Autodesk Inventor part; units mm, degrees
ref_plane "YZ Plane" through (0, 0, 0) normal (1, 0, 0) x (0, 1, 0)
ref_plane "XZ Plane" through (0, 0, 0) normal (0, 1, 0) x (-1, 0, 0)
ref_plane "XY Plane" through (0, 0, 0) normal (0, 0, 1) x (1, 0, 0)
sketch "Sketch1" plane through (0, 0, 0) normal (0, 0, 1) x (1, 0, 0)
  line L0 (0, 0) -> (6.35, 0)
  line L1 (6.35, 0) -> (6.35, 25.4)
  line L2 (6.35, 25.4) -> (0, 25.4)
  line L3 (0, 25.4) -> (0, 0)
  line L4 (6.35, 0) -> (6.35, -5.2605)
  line L5 (6.35, -5.2605) -> (12.7, -11.6105)
  line L6 (12.7, -11.6105) -> (12.7, -24.3105)
  arc A0 (12.7, -24.3105) -> (25.4, -24.3105) centre (19.05, -24.3105) ccw
  line L7 (25.4, -24.3105) -> (25.4, -6.35)
  line L8 (25.4, -6.35) -> (6.35, 12.7)
  dimension "d0" = 6.35
  dimension "d1" = 25.4
  dimension "d2" = 6.35
  dimension "d3" = 12.7
  dimension "d4" = 12.7
  dimension "d5" = 45
extrude "Extrusion1" add sketch "Sketch1" along normal blind 6.35
fillet "Fillet1" radius 3.175 1 edges at (6.35, -5.2605, 3.175)
fillet "Fillet2" radius 12.7 3 edges at (12.7, -11.6105, 3.175) (25.4, -6.35, 3.175) (6.35, 12.7, 3.175)
sketch "Sketch2" plane through (0, 0, 6.35) normal (0, 0, 1) x (1, 0, 0)
  arc A0 (12.7, -24.3105) -> (25.4, -24.3105) centre (19.05, -24.3105) ccw
hole "Hole1" at (19.05, -24.3105, 6.35) direction (0, 0, -1) diameter 6.7564 end through all
ref_plane "Work Plane1" through (11.7701, -1.7003, 6.35) normal (-0.7071, -0.7071, 0) x (-0.7071, 0.7071, 0)
properties part number "Mirror"
Work out the finished part from the listing and answer in its coordinate system (mm). A direction names the side the tool comes from. Coordinates: 2 decimals unless noted, no trailing zeros. Write each loop counter-clockwise with the first axis right and the second up, starting at its lowest first coordinate (ties: lowest second). Pieces come first, ordered by that corner, then holes.
1. Consider line 1 along Y through (x, z) = (19.05, 4.75); line 2 along Y through (x, z) = (20, 5); line 3 along X through (y, z) = (-17, 2). Determine where each line is inside the solid, lowest interval first.
Results list:
line 1: y = -30.66 to -27.69, -20.93 to 0
line 2: y = -30.59 to -27.55, -21.07 to -0.95
line 3: x = 12.7 to 25.4
2. For faces 4 (the flat face through (6.35, 22, 3)), 5 (the flat face through (13, -2, 6.35)), 6 (the flat face through (6.35, -2, 3)), determine the directions among +Z, -Z, +X, -X, +Y, -Y from which every point of the face is accessible in a straight line to the end or side of a thin tool.
Results list:
face 4: +Z, -Z, +X, +Y
face 5: +Z, +X, -X, +Y, -Y
face 6: +Z, -Z, -X, -Y
3. Flat-ended cylindrical pins translate along their axes: pin 1 (3 mm diameter, centred on x = 13.5, z = 0.5, fed in from -Y); pin 2 (1 mm diameter, centred on x = 8.5, z = 3, fed in from -Y); pin 3 (1.9 mm diameter, centred on x = 3.5, z = 4.5, fed in from -Y). Find the tip coordinate at first contact, or state that the pin passes through.
Results list:
pin 1: stops at y = -29.2
pin 2: stops at y = -7.91
pin 3: stops at y = 0
4. The part is cut by section C-C, the plane y = -18.5. Write down the section's boundary in (x, z), and give its area (3 significant figures).
Results list:
outline: (12.7, 0) - (25.4, 0) - (25.4, 6.35) - (12.7, 6.35) - close
area: 80.6 mm2
5. The part is cut by section D-D, the plane x = 5.5. Write down the section's boundary in (y, z), and give its area (3 significant figures).
Results list:
outline: (0, 0) - (25.4, 0) - (25.4, 6.35) - (0, 6.35) - close
area: 161 mm2
6. For a pull along Y with two mould halves and no side action, classify faces 1 (the flat face through (15.96, 3.09, 3.13)), 2 (the cylindrical face through (6.585, -5.144, 3.219)), 3 (the cylindrical face through (15.7, -23.87, 3.13)) as +Y half, -Y half, draft (parallel to the pull), parting line (faces both ways), or undercut.
Results list:
face 1: +Y half
face 2: -Y half
face 3: undercut
